```python
from build123d import *

# Parameters (mm, degrees)
BOSS_EXTRUDE2_DEPTH = 10
SKETCH3_R           = 45
BOSS_EXTRUDE3_DEPTH = 70
SKETCH5_W           = 40
SKETCH5_H           = 22.516210705
CUT_EXTRUDE1_DEPTH  = 40
SKETCH6_W           = 8.00117247
SKETCH6_H           = 22.516210705
SKETCH6_W_2         = 8.041819545
BOSS_EXTRUDE4_DEPTH = 32
SKETCH8_R           = 0.656937265
SKETCH8_R_2         = 0.65
CUT_EXTRUDE2_DEPTH  = 6
SHELL16_START       = 10
SHELL16_DEPTH       = 60
SHELL16_2_DEPTH     = 20
SHELL16_START_2     = 30
SHELL16_3_OUTLINE_W = 8.041819545
SHELL16_3_OUTLINE_H = 42.516210705
SHELL16_3_DEPTH     = 26
SHELL16_START_3     = 56
SHELL16_4_DEPTH     = 6
SKETCH9_R           = 2.85
CUT_EXTRUDE3_DEPTH  = 6
SKETCH10_R          = 3.25
BOSS_EXTRUDE5_DEPTH = 45


# Read off the part's stored shape, not the designer's step: Shell16
with BuildPart() as part:
    # Sketch2 → Boss-Extrude2 (new body)
    with BuildSketch(Plane(origin=(0, 0, 0), x_dir=(1, 0, 0), z_dir=(0, 1, 0))):
        with BuildLine():
            Line((-54.435630286, 55.212655463), (54.435630286, 55.212655463))
            ThreePointArc((54.435630286, 55.212655463), (68.577765909, 49.354791087), (74.435630286, 35.212655463))
            Line((74.435630286, 35.212655463), (74.435630286, -35.212655463))
            ThreePointArc((74.435630286, -35.212655463), (68.577765909, -49.354791087), (54.435630286, -55.212655463))
            Line((54.435630286, -55.212655463), (-54.435630286, -55.212655463))
            ThreePointArc((-54.435630286, -55.212655463), (-68.577765909, -49.354791087), (-74.435630286, -35.212655463))
            Line((-74.435630286, -35.212655463), (-74.435630286, 35.212655463))
            ThreePointArc((-74.435630286, 35.212655463), (-68.577765909, 49.354791087), (-54.435630286, 55.212655463))
        make_face()
    extrude(amount=BOSS_EXTRUDE2_DEPTH)

    # Sketch3 → Boss-Extrude3 (add)
    with BuildSketch(Plane(origin=(0, 10, 0), x_dir=(1, 0, 0), z_dir=(0, 1, 0))):
        with Locations(Location((0, 0, 0), (0, 0, 270))):
            Circle(SKETCH3_R)
    extrude(amount=BOSS_EXTRUDE3_DEPTH)

    # Sketch5 → Cut-Extrude1 (cut)
    with BuildSketch(Plane(origin=(0, 80, 0), x_dir=(1, 0, 0), z_dir=(0, 1, 0))):
        with Locations((-18.795917007, -0.647948509)):
            Rectangle(SKETCH5_W, SKETCH5_H)
    extrude(amount=-CUT_EXTRUDE1_DEPTH, mode=Mode.SUBTRACT)

    # Sketch6 → Boss-Extrude4 (add)
    with BuildSketch(Plane(origin=(0, 40, 0), x_dir=(1, 0, 0), z_dir=(0, 1, 0))):
        with Locations((-34.795330772, -0.647948509)):
            Rectangle(SKETCH6_W, SKETCH6_H)
        with Locations((-2.81682678, -0.647948509)):
            Rectangle(SKETCH6_W_2, SKETCH6_H)
    extrude(amount=BOSS_EXTRUDE4_DEPTH)

    # Sketch8 → Cut-Extrude2 (cut)
    with BuildSketch(Plane(origin=(0, 72, 0), x_dir=(1, 0, 0), z_dir=(0, 1, 0))):
        with Locations(Location((-3.150273661, 6.373412823, 0), (0, 0, 270))):
            Circle(SKETCH8_R)
        with Locations(Location((-3.150273661, -7.089946011, 0), (0, 0, 270))):
            Circle(SKETCH8_R_2)
        with Locations(Location((-34.990160193, 6.373412823, 0), (0, 0, 270))):
            Circle(SKETCH8_R_2)
        with Locations(Location((-34.990160193, -7.089946011, 0), (0, 0, 270))):
            Circle(SKETCH8_R_2)
    extrude(amount=-CUT_EXTRUDE2_DEPTH, mode=Mode.SUBTRACT)

    # Shell16 outline → Shell16 (cut)
    with BuildSketch(Plane(origin=(0, 0, 0), x_dir=(1, 0, 0), z_dir=(0, 1, 0)).offset(SHELL16_START)):
        with BuildLine():
            ThreePointArc((-27.296974268, -21.906053862), (34.990492106, 0.815758643), (-28.28818543, 20.610156843))
            Line((-28.28818543, 20.610156843), (11.204082993, 20.610156843))
            Line((11.204082993, 20.610156843), (11.204082993, -21.906053862))
            Line((11.204082993, -21.906053862), (-27.296974268, -21.906053862))
        make_face()
    extrude(amount=SHELL16_DEPTH, mode=Mode.SUBTRACT)

    # Shell16 2 outline → Shell16 2 (cut)
    with BuildSketch(Plane(origin=(0, 0, 0), x_dir=(1, 0, 0), z_dir=(0, 1, 0)).offset(SHELL16_START)):
        with BuildLine():
            ThreePointArc((-28.28818543, 20.610156843), (-34.990492106, -0.815758643), (-27.296974268, -21.906053862))
            Line((-27.296974268, -21.906053862), (11.204082993, -21.906053862))
            Line((11.204082993, -21.906053862), (11.204082993, 20.610156843))
            Line((11.204082993, 20.610156843), (-28.28818543, 20.610156843))
        make_face()
    extrude(amount=SHELL16_2_DEPTH, mode=Mode.SUBTRACT)

    # Shell16 3 outline → Shell16 3 (cut)
    with BuildSketch(Plane(origin=(0, 0, 0), x_dir=(1, 0, 0), z_dir=(0, 1, 0)).offset(SHELL16_START_2)):
        with Locations((7.183173221, -0.647948509)):
            Rectangle(SHELL16_3_OUTLINE_W, SHELL16_3_OUTLINE_H)
    extrude(amount=SHELL16_3_DEPTH, mode=Mode.SUBTRACT)

    # Shell16 4 outline → Shell16 4 (cut)
    with BuildSketch(Plane(origin=(0, 0, 0), x_dir=(1, 0, 0), z_dir=(0, 1, 0)).offset(SHELL16_START_3)):
        with BuildLine():
            Line((11.204082993, 20.610156843), (3.162263448, 20.610156843))
            Line((3.162263448, 20.610156843), (3.162263448, 14.95957536))
            ThreePointArc((3.162263448, 14.95957536), (7.421869806, 7.715088784), (5.106897043, -0.363756008))
            ThreePointArc((5.106897043, -0.363756008), (7.414773238, -8.432437732), (3.162263448, -15.667496667))
            Line((3.162263448, -15.667496667), (3.162263448, -21.906053862))
            Line((3.162263448, -21.906053862), (11.204082993, -21.906053862))
            Line((11.204082993, -21.906053862), (11.204082993, 20.610156843))
        make_face()
    extrude(amount=SHELL16_4_DEPTH, mode=Mode.SUBTRACT)

    # Sketch9 → Cut-Extrude3 (cut)
    with BuildSketch(Plane(origin=(0, 10, 0), x_dir=(1, 0, 0), z_dir=(0, 1, 0))):
        with Locations(Location((-64.63637004, 43.938587161, 0), (0, 0, 270))):
            Circle(SKETCH9_R)
        with Locations(Location((63.260769817, 43.938587161, 0), (0, 0, 270))):
            Circle(SKETCH9_R)
        with Locations(Location((-64.63637004, -46.106335294, 0), (0, 0, 270))):
            Circle(SKETCH9_R)
        with Locations(Location((63.260769817, -46.106335294, 0), (0, 0, 270))):
            Circle(SKETCH9_R)
    extrude(amount=-CUT_EXTRUDE3_DEPTH, mode=Mode.SUBTRACT)

    # Sketch10 → Boss-Extrude5 (add)
    with BuildSketch(Plane(origin=(0, 40, 0), x_dir=(1, 0, 0), z_dir=(0, 1, 0))):
        with Locations(Location((-11.127628751, -0.64794851, 0), (0, 0, 270))):
            Circle(SKETCH10_R)
    extrude(amount=BOSS_EXTRUDE5_DEPTH)


solid = part.part
```
Design review of the part built by this model. Coordinates are the model's own, in mm. A direction names the side the tool comes from. Give positions to 0.01 mm unless a question says otherwise; leave off trailing zeros. Loops run counter-clockwise (first coordinate to the right, second up) from the corner with the lowest first, then second, coordinate; pieces in that order, holes last. Notation, with made-up numbers: M 32.25,-0.75 L 50.25,-0.75 A33 ccw 50.25,37.25 Z; hole C 78,38.25 d3. An arc over 180 degrees is marked long. Return JSON: item names as keys, results as strings. Group by question number.
Item 1: Tool access review of faces 1 (the cylindrical face through (7.43, 58.96, 8.31)), 2 (the cylindrical face through (68.73, 4.93, 49.2)), 3 (the flat face through (63, 4, 46)): name each direction out of +Z, -Z, +X, -X, +Y, -Y from which nothing blocks a thin tool from reaching the whole face with its end or side.
Item 2: Mouldability with a two-part tool opening along Y and no side actions: class faces 4 (the flat face through (3.162, 42, 0)), 5 (the flat face through (34, 10, -38)), 6 (the flat face through (1, 0, -1)) as released by +Y, released by -Y, zero draft, split by the parting line, or undercut.
Item 3: We need section B-B (z = 18.5). Give the boundary of the cut face in (x, y).
Item 4: We need section A-A (y = 60). Give the boundary of the cut face in (x, z), and give its area (3 significant figures).
Item 5: We need section D-D (x = -42). Give the boundary of the cut face in (y, z).
Item 6: We need section C-C (x = 26.5). Give the boundary of the cut face in (y, z).
Item 7: For probe 1 along X at (y, z) = (24.5, -1.5) (3 decimals); probe 2 along Z at (x, y) = (-22.5, 51); probe 3 along Y at (x, z) = (-2, -8.5), list the stretches that pass through material, from the lowest coordinate up.
Item 8: Insertion check: pin 1 Ø10 at (x, y) = (11.5, 68.5) entering from -Z; pin 2 Ø18 at (y, z) = (62, 1) entering from -X; pin 3 Ø2 at (x, y) = (-34, 72) entering from -Z. Each pin has a flat end and moves straight along its axis. Give the tip position at first contact, or say it passes through.
Output:
{
 "1": {"face 1": "none", "face 2": "+Z, +X, +Y, -Y", "face 3": "+Y"},
 "2": {"face 4": "undercut", "face 5": "released by +Y", "face 6": "released by -Y"},
 "3": {"outline": "M -74.44,0 L 74.44,0 L 74.44,10 L 41.02,10 L 41.02,80 L -41.02,80 L -41.02,10 L -74.44,10 Z; hole M -29.71,10 L 29.71,10 L 29.71,70 L 11.2,70 L 11.2,62 L 3.16,62 L 3.16,30 L -29.71,30 Z"},
 "4": {"outline": "C 0,0 d90; C -11.13,0.65 d6.5; hole M -30.79,-10.61 L -6.84,-10.61 L -6.84,11.91 L -30.79,11.91 Z; hole M -28.29,-20.61 A35 ccw long -27.3,21.91 L 3.16,21.91 L 3.16,15.67 A10.65 cw 5.11,0.36 A10.66 cw 3.16,-14.96 L 3.16,-20.61 Z", "area": "3,630 mm^2"},
 "5": {"outline": "M 0,-55.21 L 10,-55.21 L 10,-16.16 L 80,-16.16 L 80,16.16 L 10,16.16 L 10,55.21 L 0,55.21 Z"},
 "6": {"outline": "M 0,-55.21 L 10,-55.21 L 10,-36.37 L 80,-36.37 L 80,36.37 L 10,36.37 L 10,55.21 L 0,55.21 Z; hole M 10,-22.86 L 70,-22.86 L 70,22.86 L 10,22.86 Z"},
 "7": {"probe 1": "x = -44.975 to -34.968, 34.968 to 44.975", "probe 2": "z = -38.97 to -26.81, -20.61 to -10.61, 11.91 to 21.91, 26.81 to 38.97", "probe 3": "y = 0 to 10, 30 to 72"},
 "8": {"pin 1": "stops at z = -44.53", "pin 2": "stops at x = -45", "pin 3": "stops at z = -30.59"}
}
